The listing builds one solid part. Answer for the finished solid, in the listing's coordinates (mm). Face numbers are marked on the shaded views. A direction names the side the tool comes from. Coordinates: 2 decimals unless noted, no trailing zeros. Order: outer loops, then holes, each group sorted by start corner. A loop starts at its lowest first (then second) coordinate and runs counter-clockwise, first axis right, second up. Notation, with made-up numbers: (70.5, -21.5) - (97.5, -21.5) arc R29 cw to (97.5, 4.5) - close; hole circle Ø8 at (-4.5, 74.25). An arc over 180 degrees is marked (long way). Use one line per item in the form item = value. Start each with the question number.
Item 1: Each of these flat-tipped pins is pushed along its axis until it touches: pin 1 Ø0.7 at (y, z) = (4, 0.5) entering from -X; pin 2 Ø1 at (x, y) = (1, 2.5) entering from -Z; pin 3 Ø3.5 at (x, y) = (3, 3.5) entering from +Z; pin 4 Ø1.5 at (x, y) = (2.5, 4.5) entering from +Z. Where does it stop, or does it pass through?
Item 2: Consider line 1 along X through (y, z) = (1.5, 1.15); line 2 along X through (y, z) = (4.35, 0.55); line 3 along Z through (x, y) = (5.75, 6). Determine where each line is inside the solid, lowest interval first. Write a range as [from, to].
Item 3: A tool of negligible diameter and unlimited length cuts with its end or side. For the marked faces 5, 6, 7, 8 and 9, from which of +Z, -Z, +X, -X, +Y, -Y can it reach the whole face along a straight path? Write none if from no direction.
Item 4: Section A-A, the plane y = 4.35 is taken. Write down the section's boundary in (x, z), and give its area (3 significant figures).
Item 5: Section C-C, the plane z = 0.5 is taken. Write down the section's boundary in (x, y), and give its area (3 significant figures).
Item 6: The mould has two halves that part along X. Classify the marked faces 1, 2, 3 and 4: released by +X, released by -X, zero draft, split by the parting line, or undercut.
Item 7: Section D-D, the plane y = 2.75 is taken. Write down the section's boundary in (x, z).
Item 8: Section B-B, the plane x = 3.2 is taken. Write down the section's boundary in (y, z), and give its area (3 significant figures).
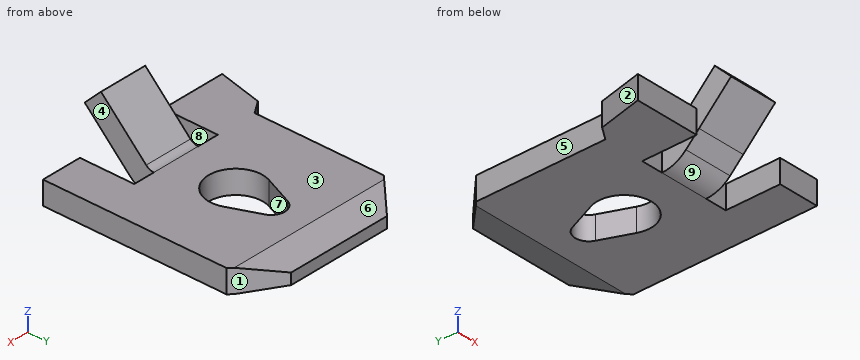
from build123d import *

# Parameters (mm, degrees)
BOSS_EXTRUDE1_DEPTH    = 6.4
CUT_EXTRUDE1_REACH     = 12.397
CUT_EXTRUDE2_DEPTH     = 0.85
SKETCH6_W              = 0.8
SKETCH6_H              = 2
CUT_EXTRUDE3_DEPTH     = 0.85
SKETCH7_W              = 1.8
SKETCH7_H              = 0.85
BOSS_EXTRUDE2_DEPTH    = 1
SKETCHED_START         = 2.3
SKETCHED_BEND1_DEPTH   = 1.8
SKETCHED_BEND1_2_DEPTH = 1.8
BOSS_EXTRUDE3_DEPTH    = 0.85


# Read off the part's stored shape, not the designer's step: Sketched Bend1
with BuildPart() as part:
    # Sketch1 → Boss-Extrude1 (new body)
    with BuildSketch(Plane(origin=(0, 0, 0), x_dir=(0, 0, -1), z_dir=(1, 0, 0))):
        Polygon((0, 0.15), (0, 7.05), (-0.241393443, 8.15), (-0.647131148, 8.15), (-0.85, 7.05), (-0.85, 0.15), align=None)
    extrude(amount=BOSS_EXTRUDE1_DEPTH)

    # Cut-Extrude1: up to this face of the body (flat: up to its plane)
    cut_extrude1_end = Plane(part.part.faces().sort_by_distance((3.2, 3.6, 0))[0])
    # Sketch4 → Cut-Extrude1 (cut, up to the picked face)
    with BuildSketch(Plane.XY.offset(0.85), mode=Mode.PRIVATE) as cut_extrude1_sk1:
        Polygon((0, 6.9), (1.25, 8.15), (0, 8.15), align=None)
    cut_extrude1_tool1 = split(extrude(cut_extrude1_sk1.sketch, amount=-CUT_EXTRUDE1_REACH, mode=Mode.PRIVATE), bisect_by=cut_extrude1_end, keep=Keep.BOTH, mode=Mode.PRIVATE)
    # Sketch4 → Cut-Extrude1 (cut, up to the picked face)
    with BuildSketch(Plane.XY.offset(0.85), mode=Mode.PRIVATE) as cut_extrude1_sk2:
        Polygon((5.15, 8.15), (6.4, 6.9), (6.4, 8.15), align=None)
    cut_extrude1_tool2 = split(extrude(cut_extrude1_sk2.sketch, amount=-CUT_EXTRUDE1_REACH, mode=Mode.PRIVATE), bisect_by=cut_extrude1_end, keep=Keep.BOTH, mode=Mode.PRIVATE)
    add(cut_extrude1_tool1.solids().sort_by(Axis((0.416667, 7.733333, 0.85), (0, 0, -1)))[0], mode=Mode.SUBTRACT)
    add(cut_extrude1_tool2.solids().sort_by(Axis((5.983333, 7.733333, 0.85), (0, 0, -1)))[0], mode=Mode.SUBTRACT)

    # Sketch5 → Cut-Extrude2 (cut)
    with BuildSketch(Plane.XY.offset(0.85)):
        with BuildLine():
            Line((2.738461538, 5.842307692), (2.276923077, 4.734615385))
            ThreePointArc((2.276923077, 4.734615385), (3.20010742, 3.350000006), (4.122994271, 4.734813689))
            Line((4.122994271, 4.734813689), (3.667436975, 5.827489929))
            ThreePointArc((3.667436975, 5.827489929), (3.207974312, 6.149936406), (2.738461538, 5.842307692))
        make_face()
    extrude(amount=-CUT_EXTRUDE2_DEPTH, mode=Mode.SUBTRACT)

    # Sketch6 → Cut-Extrude3 (cut)
    with BuildSketch(Plane(origin=(0, 0, 0), x_dir=(-1, 0, 0), z_dir=(0, 0, -1))):
        with Locations((-4.5, 1.15)):
            Rectangle(SKETCH6_W, SKETCH6_H)
        with Locations((-1.9, 1.15)):
            Rectangle(SKETCH6_W, SKETCH6_H)
    extrude(amount=-CUT_EXTRUDE3_DEPTH, mode=Mode.SUBTRACT)

    # Sketch7 → Boss-Extrude2 (add)
    with BuildSketch(Plane.XZ.offset(-0.15)):
        with Locations((3.2, 0.425)):
            Rectangle(SKETCH7_W, SKETCH7_H)
    extrude(amount=BOSS_EXTRUDE2_DEPTH)

    # Sketched Bend1 outline → Sketched Bend1 (cut)
    with BuildSketch(Plane.YZ.offset(SKETCHED_START)):
        with BuildLine():
            Line((1.266116524, 0.366116524), (0.782233048, 0.85))
            Line((0.782233048, 0.85), (-0.85, 0.85))
            Line((-0.85, 0.85), (-0.85, 0))
            Line((-0.85, 0), (2.15, 0))
            ThreePointArc((2.15, 0), (1.67164571, 0.095150584), (1.266116524, 0.366116524))
        make_face()
    extrude(amount=SKETCHED_BEND1_DEPTH, mode=Mode.SUBTRACT)

    # Sketched Bend1 2 outline → Sketched Bend1 2 (add)
    with BuildSketch(Plane.YZ.offset(SKETCHED_START)):
        with BuildLine():
            ThreePointArc((2.15, 0.85), (1.996926627, 0.880448187), (1.867157288, 0.967157288))
            Line((1.867157288, 0.967157288), (0.204009247, 2.630305328))
            Line((0.204009247, 2.630305328), (-0.397031517, 2.029264564))
            Line((-0.397031517, 2.029264564), (0.782233048, 0.85))
            Line((0.782233048, 0.85), (2.15, 0.85))
        make_face()
    extrude(amount=SKETCHED_BEND1_2_DEPTH)

    # Sketch15 → Boss-Extrude3 (add)
    with BuildSketch(Plane.XY.offset(0.85)):
        Polygon((0, 2.15), (-0.50789834, 1.808617859), (-0.890356386, 0.15), (0, 0.15), align=None)
    extrude(amount=-BOSS_EXTRUDE3_DEPTH)


solid = part.part
Response:
q1.pin_1 = 0
q1.pin_2 = 0
q1.pin_3 = 1.08
q1.pin_4 = 0.85
q2.line_1 = [2.3, 4.1]
q2.line_2 = [0, 2.2], [4.2, 6.4]
q2.line_3 = [0, 0.85]
q3.face_5 = +Z, -Z, -X, +Y
q3.face_6 = +Z, +X, -X, +Y
q3.face_7 = +Z, -Z
q3.face_8 = +Z, -Z, -Y
q3.face_9 = -Z, -Y
q4.outline = (0, 0) - (2.2, 0) - (2.2, 0.85) - (0, 0.85) - close; (4.2, 0) - (6.4, 0) - (6.4, 0.85) - (4.2, 0.85) - close
q4.area = 3.74 mm2
q5.outline = (-0.89, 0.15) - (1.5, 0.15) - (1.5, 2.15) - (2.3, 2.15) - (2.3, 1.13) - (4.1, 1.13) - (4.1, 2.15) - (4.9, 2.15) - (4.9, 0.15) - (6.4, 0.15) - (6.4, 6.9) - (5.15, 8.15) - (1.25, 8.15) - (0, 6.9) - (0, 2.15) - (-0.51, 1.81) - close; hole (2.28, 4.73) arc R1 ccw (long way) to (4.12, 4.73) - (3.67, 5.83) arc R0.5 ccw to (2.74, 5.84) - close
q5.area = 41.9 mm2
q6.face_1 = released by +X
q6.face_2 = released by -X
q6.face_3 = zero draft
q6.face_4 = undercut
q7.outline = (0, 0) - (6.4, 0) - (6.4, 0.85) - (0, 0.85) - close
q8.outline = (-0.4, 2.03) - (1.27, 0.37) arc R1.25 ccw to (2.15, 0) - (3.35, 0) - (3.35, 0.85) - (2.15, 0.85) arc R0.4 cw to (1.87, 0.97) - (0.2, 2.63) - close; (6.15, 0) - (7.05, 0) - (8.15, 0.24) - (8.15, 0.65) - (7.05, 0.85) - (6.15, 0.85) - close
q8.area = 5.03 mm2
